The model under review builds one solid part; all positions refer to its coordinate system, in mm. A direction names the side the tool comes from. Round coordinates to 2 decimals unless told otherwise and drop trailing zeros. Loops run counter-clockwise (first coordinate to the right, second up) from the corner with the lowest first, then second, coordinate; pieces in that order, holes last. Notation, with made-up numbers: M -36.5,27 L -26.5,27 A20 cw -26.5,60 Z; hole C 9,88 d7. An arc over 180 degrees is marked long. Return JSON: item names as keys, results as strings. Group by question number.
Q1. Clearance check with flat-ended pins moving along their axes: pin 1 Ø4 at (x, z) = (11, 17) entering from -Y; pin 2 Ø3 at (x, y) = (4.5, 1) entering from -Z; pin 3 Ø2 at (y, z) = (5, -0.5) entering from -X; pin 4 Ø1.4 at (x, z) = (4, -1) entering from -Y. State where each tip first meets the part, or that it passes through.
Q2. Consider section C-C (x = 15.75). State the section outline as (y, z) points, and give its area (3 significant figures).
Q3. Draft analysis for pull direction Y (two halves, no side actions). For faces 5 (the face through (1.5, 5.1, 27.4)), 6 (the face through (5, 0, 58)), 7 (the face through (0, 5, 57)), state which applies: pulls with the +Y half, pulls with the -Y half, needs draft (parallel to the pull), parting line crosses it, or undercut.
Q4. To check wall thickness, follow line 1 along Y through (x, z) = (0.7, 30); line 2 along X through (y, z) = (7.5, 17.5); line 3 along Z through (x, y) = (15.5, 1.25). State the ranges of each line that lie inside material, in increasing order.
Q5. Consider section D-D (z = 18). State the section outline as (x, y) points, and give its area (3 significant figures).
Q6. Consider section A-A (y = 5). State the section outline as (x, z) points.
Q7. Consider section B-B (z = 30). State the section outline as (x, y) points.
Q8. For faces 1 (the face through (4, 3.1, -1)), 2 (the face through (3, 5, 30)), 3 (the face through (4, 6.9, -1)), 4 (the face through (14, 5, 107)), list the 3-axis set-ups (+Z, -Z, +X, -X, +Y, -Y) from which the entire face can be reached by the end or side of a thin tool; tool diameter is ignored.
from build123d import *

# Parameters (mm, degrees)
SKETCH1_W           = 8
SKETCH1_H           = 10
BOSS_EXTRUDE1_DEPTH = 115
SKETCH2_W           = 3.8
SKETCH2_H           = 3.8
BOSS_EXTRUDE2_DEPTH = 1.8
SKETCH4_W           = 8
SKETCH4_H           = 10
BOSS_EXTRUDE4_DEPTH = 12
SKETCH5_R           = 2.6
CUT_EXTRUDE1_DEPTH  = 3


with BuildPart() as part:
    # Sketch1 → Boss-Extrude1 (new body)
    with BuildSketch(Plane.XY):
        with Locations((4, 5)):
            Rectangle(SKETCH1_W, SKETCH1_H)
    extrude(amount=BOSS_EXTRUDE1_DEPTH)

    # Sketch2 → Boss-Extrude2 (add)
    with BuildSketch(Plane(origin=(0, 0, 0), x_dir=(-1, 0, 0), z_dir=(0, 0, -1))):
        with Locations((-4, 5)):
            Rectangle(SKETCH2_W, SKETCH2_H)
    extrude(amount=BOSS_EXTRUDE2_DEPTH)

    # Sketch4 → Boss-Extrude4 (add)
    with BuildSketch(Plane(origin=(8, 0, 0), x_dir=(0, 0, -1), z_dir=(1, 0, 0))):
        with Locations((-111, 5)):
            Rectangle(SKETCH4_W, SKETCH4_H)
    extrude(amount=BOSS_EXTRUDE4_DEPTH)

    # Sketch5 → Cut-Extrude1 (cut)
    with BuildSketch(Plane.ZY):
        with Locations((30, 5)):
            Circle(SKETCH5_R)
    extrude(amount=-CUT_EXTRUDE1_DEPTH, mode=Mode.SUBTRACT)


solid = part.part
Values:
{
 "1": {"pin 1": "passes through", "pin 2": "stops at z = 0", "pin 3": "stops at x = 0", "pin 4": "stops at y = 3.1"},
 "2": {"outline": "M 0,107 L 10,107 L 10,115 L 0,115 Z", "area": "80.0 mm2"},
 "3": {"face 5": "undercut", "face 6": "pulls with the -Y half", "face 7": "needs draft"},
 "4": {"line 1": "y = 0 to 2.4, 7.6 to 10", "line 2": "x = 0 to 8", "line 3": "z = 107 to 115"},
 "5": {"outline": "M 0,0 L 8,0 L 8,10 L 0,10 Z", "area": "80.0 mm2"},
 "6": {"outline": "M 0,0 L 2.1,0 L 2.1,-1.8 L 5.9,-1.8 L 5.9,0 L 8,0 L 8,107 L 20,107 L 20,115 L 0,115 L 0,32.6 L 3,32.6 L 3,27.4 L 0,27.4 Z"},
 "7": {"outline": "M 0,0 L 8,0 L 8,10 L 0,10 L 0,7.6 L 3,7.6 L 3,2.4 L 0,2.4 Z"},
 "8": {"face 1": "-Z, +X, -X, -Y", "face 2": "-X", "face 3": "-Z, +X, -X, +Y", "face 4": "-Z, +X, +Y, -Y"}
}
